Input: part model. Units: mm. Frame: model coordinates. A direction names the side the tool comes from. Round coordinates to 2 decimals unless told otherwise and drop trailing zeros. Loops run counter-clockwise (first coordinate to the right, second up) from the corner with the lowest first, then second, coordinate; pieces in that order, holes last. Notation, with made-up numbers: (11, -28.5) -> (26, -28.5) arc R14 cw to (26, -17.5) -> close; hole circle Ø11 at (46.5, 85). An arc over 180 degrees is marked (long way). Answer as a JSON object with one key per item and string values. Group by question number.
Item 1: Section query C-C on z = 455. Return loops of the section in (x, y), and give its area (3 significant figures).
Item 2: Section query A-A on y = -154. Return loops of the section in (x, z).
Item 3: Set-up query: faces 1 (the flat face through (0, 38, 279)), 2 (the flat face through (222, 216.106, 311)). Return all of +Z, -Z, +X, -X, +Y, -Y with unobstructed straight access to the full face (end or side cutting, diameter ignored); none if empty.
Item 4: Draft query along Z for faces 3 (the flat face through (228, 19, 209.82)), 4 (the flat face through (222, -149, -0.18)), 5 (the flat face through (222, -183.894, 218)), 6 (the flat face through (420, 13, 459)). Return one class per face: released by +Z, released by -Z, zero draft, split by the parting line, or undercut.
Item 5: Section query D-D on y = 103. Return loops of the section in (x, z).
Item 6: Pin query (flat end, axial travel): pin 1 (5 mm diameter, centred on x = 267, z = 378.5, fed in from -Y). Return the tip coordinate at first contact, or that it passes through.
Item 7: Material intervals for line 1 (Z direction, x = 115.5, y = -122.5); line 2 (Z direction, x = 191.5, y = 35.5); line 3 (X direction, y = 9.5, z = 205.5), sorted ascending. Write a range as [from, to].
Item 8: Section query B-B on x = 231.5. Return loops of the section in (y, z), and give its area (3 significant figures).
from build123d import *

# Parameters (mm, degrees)
F1_DEPTH = 450
F2_W     = 390
F2_H     = 470
F3_DEPTH = 400
F4_W     = 400
F4_H     = 25
F5_DEPTH = 390
F6_W     = 400
F6_H     = 25
F7_DEPTH = 390


with BuildPart() as f1:
    # F0 (on Right) → F1 (new body)
    with BuildSketch(Plane.YZ):
        with BuildLine():
            Line((266.10621, -0.179865), (266.10621, 549.820135))
            Line((266.10621, 549.820135), (-183.89379, 549.820135))
            Line((-183.89379, 549.820135), (-183.89379, -0.179865))
            Line((-183.89379, -0.179865), (-113.89379, -0.179865))
            ThreePointArc((-113.89379, -0.179865), (41.10621, 39.031723), (196.10621, -0.179865))
            Line((196.10621, -0.179865), (266.10621, -0.179865))
        make_face()
    extrude(amount=F1_DEPTH)

    # F2 (on face) → F3 (cut)
    with BuildSketch(Plane.XZ.offset(183.89379)):
        with Locations((225, 274.820135)):
            Rectangle(F2_W, F2_H)
    extrude(amount=-F3_DEPTH, mode=Mode.SUBTRACT)

    # F4 (on face) → F5 (join)
    with BuildSketch(Plane(origin=(420, 0, 0), x_dir=(0, -1, 0), z_dir=(-1, 0, 0))):
        with Locations((-16.10621, 397.320135)):
            Rectangle(F4_W, F4_H)
    extrude(amount=F5_DEPTH)

    # F6 (on face) → F7 (join)
    with BuildSketch(Plane(origin=(420, 0, 0), x_dir=(0, -1, 0), z_dir=(-1, 0, 0))):
        with Locations((-16.10621, 222.320135)):
            Rectangle(F6_W, F6_H)
    extrude(amount=F7_DEPTH)


solid = f1.part
Solved:
{
 "1": {"outline": "(0, -183.89) -> (30, -183.89) -> (30, 216.11) -> (420, 216.11) -> (420, -183.89) -> (450, -183.89) -> (450, 266.11) -> (0, 266.11) -> close", "area": "46,500 mm²"},
 "2": {"outline": "(0, -0.18) -> (450, -0.18) -> (450, 549.82) -> (0, 549.82) -> close; hole (30, 39.82) -> (420, 39.82) -> (420, 209.82) -> (30, 209.82) -> close; hole (30, 234.82) -> (420, 234.82) -> (420, 384.82) -> (30, 384.82) -> close; hole (30, 409.82) -> (420, 409.82) -> (420, 509.82) -> (30, 509.82) -> close"},
 "3": {"face 1": "+Z, -Z, -X, +Y, -Y", "face 2": "-Y"},
 "4": {"face 3": "undercut", "face 4": "released by -Z", "face 5": "zero draft", "face 6": "undercut"},
 "5": {"outline": "(0, 33.1) -> (450, 33.1) -> (450, 549.82) -> (0, 549.82) -> close; hole (30, 39.82) -> (420, 39.82) -> (420, 209.82) -> (30, 209.82) -> close; hole (30, 234.82) -> (420, 234.82) -> (420, 384.82) -> (30, 384.82) -> close; hole (30, 409.82) -> (420, 409.82) -> (420, 509.82) -> (30, 509.82) -> close"},
 "6": {"pin 1": "y = 216.11"},
 "7": {"line 1": "[-0.18, 39.82], [209.82, 234.82], [384.82, 409.82], [509.82, 549.82]", "line 2": "[38.98, 39.82], [209.82, 234.82], [384.82, 409.82], [509.82, 549.82]", "line 3": "[0, 30], [420, 450]"},
 "8": {"outline": "(-183.89, -0.18) -> (-113.89, -0.18) arc R325.96 cw to (196.11, -0.18) -> (266.11, -0.18) -> (266.11, 549.82) -> (-183.89, 549.82) -> (-183.89, 509.82) -> (216.11, 509.82) -> (216.11, 409.82) -> (-183.89, 409.82) -> (-183.89, 384.82) -> (216.11, 384.82) -> (216.11, 234.82) -> (-183.89, 234.82) -> (-183.89, 209.82) -> (216.11, 209.82) -> (216.11, 39.82) -> (-183.89, 39.82) -> close", "area": "71,300 mm²"}
}
